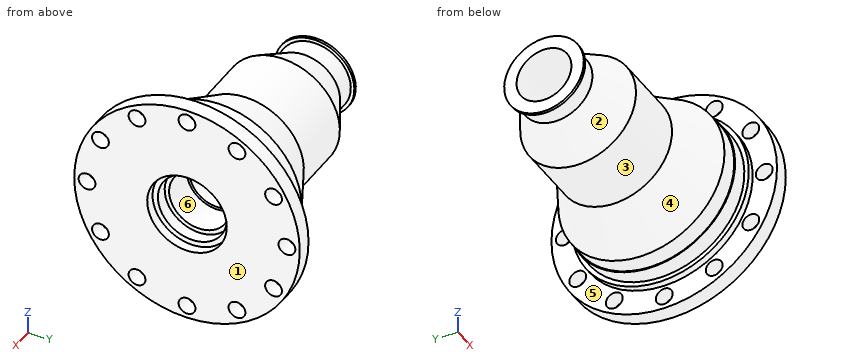
```python
from build123d import *

# Parameters (mm, degrees)
SKETCH_3_R           = 9.5
CUT_EXTRUDE_1_DEPTH  = 321.526909947
SKETCH_4_R           = 9.5
CUT_EXTRUDE_2_DEPTH  = 321.526909947
SKETCH_5_R           = 9.5
CUT_EXTRUDE_3_DEPTH  = 321.526909947
SKETCH_6_R           = 9.5
CUT_EXTRUDE_4_DEPTH  = 321.526909947
SKETCH_7_R           = 9.5
CUT_EXTRUDE_5_DEPTH  = 321.526909947
SKETCH_8_R           = 9.5
CUT_EXTRUDE_6_DEPTH  = 321.526909947
SKETCH_9_R           = 9.5
CUT_EXTRUDE_7_DEPTH  = 321.526909947
SKETCH_10_R          = 9.5
CUT_EXTRUDE_8_DEPTH  = 321.526909947
SKETCH_11_R          = 9.5
CUT_EXTRUDE_9_DEPTH  = 321.526909947
SKETCH_12_R          = 9.5
CUT_EXTRUDE_10_DEPTH = 321.526909947
SKETCH_13_R          = 9.5
CUT_EXTRUDE_11_DEPTH = 321.526909947
SKETCH_14_R          = 9.5
CUT_EXTRUDE_12_DEPTH = 321.526909947


with BuildPart() as part:
    # Эскиз1 → Повернуть1 (revolve)
    with BuildSketch(Plane.XY, mode=Mode.PRIVATE) as revolve_1_sk:
        Polygon((0, 0), (265, 0), (265, 127.5), (247, 127.5), (247, 100), (239, 100), (239, 95), (220, 95), (220, 94), (200, 94), (144, 65.5), (70, 65.5), (25, 41), (3, 41), (3, 45), (0, 45), align=None)
    revolve(revolve_1_sk.sketch.rotate(Axis((0, 0, 0), (1, 0, 0)), 90), axis=Axis((0, 0, 0), (1, 0, 0)))

    # Эскиз2 → Вырез-Повернуть1 (revolve, cut)
    with BuildSketch(Plane.XY, mode=Mode.PRIVATE) as cut_revolve_1_sk:
        Polygon((0, 0), (265, 0), (265, 45), (254, 45), (254, 39), (240, 39), (240, 34), (203.5, 34), (203.5, 31), (0, 31), align=None)
    revolve(cut_revolve_1_sk.sketch.rotate(Axis((0, 0, 0), (1, 0, 0)), 90), axis=Axis((0, 0, 0), (1, 0, 0)), mode=Mode.SUBTRACT)

    # Эскиз3 → Вырез-Вытянуть1 (cut, through all)
    with BuildSketch(Plane(origin=(0, 0, 0), x_dir=(0, 0, -1), z_dir=(1, 0, 0))):
        with Locations((0, 113)):
            Circle(SKETCH_3_R)
    extrude(amount=CUT_EXTRUDE_1_DEPTH, mode=Mode.SUBTRACT)

    # Эскиз4 → Вырез-Вытянуть2 (cut, through all)
    with BuildSketch(Plane(origin=(0, 0, 0), x_dir=(0, 0, -1), z_dir=(1, 0, 0))):
        with Locations((-56.5, 97.860870628)):
            Circle(SKETCH_4_R)
    extrude(amount=CUT_EXTRUDE_2_DEPTH, mode=Mode.SUBTRACT)

    # Эскиз5 → Вырез-Вытянуть3 (cut, through all)
    with BuildSketch(Plane(origin=(0, 0, 0), x_dir=(0, 0, -1), z_dir=(1, 0, 0))):
        with Locations((-97.860870628, 56.5)):
            Circle(SKETCH_5_R)
    extrude(amount=CUT_EXTRUDE_3_DEPTH, mode=Mode.SUBTRACT)

    # Эскиз6 → Вырез-Вытянуть4 (cut, through all)
    with BuildSketch(Plane(origin=(0, 0, 0), x_dir=(0, 0, -1), z_dir=(1, 0, 0))):
        with Locations((-113, 0)):
            Circle(SKETCH_6_R)
    extrude(amount=CUT_EXTRUDE_4_DEPTH, mode=Mode.SUBTRACT)

    # Эскиз7 → Вырез-Вытянуть5 (cut, through all)
    with BuildSketch(Plane(origin=(0, 0, 0), x_dir=(0, 0, -1), z_dir=(1, 0, 0))):
        with Locations((-97.860870628, -56.5)):
            Circle(SKETCH_7_R)
    extrude(amount=CUT_EXTRUDE_5_DEPTH, mode=Mode.SUBTRACT)

    # Эскиз8 → Вырез-Вытянуть6 (cut, through all)
    with BuildSketch(Plane(origin=(0, 0, 0), x_dir=(0, 0, -1), z_dir=(1, 0, 0))):
        with Locations((-56.5, -97.860870628)):
            Circle(SKETCH_8_R)
    extrude(amount=CUT_EXTRUDE_6_DEPTH, mode=Mode.SUBTRACT)

    # Эскиз9 → Вырез-Вытянуть7 (cut, through all)
    with BuildSketch(Plane(origin=(0, 0, 0), x_dir=(0, 0, -1), z_dir=(1, 0, 0))):
        with Locations((0, -113)):
            Circle(SKETCH_9_R)
    extrude(amount=CUT_EXTRUDE_7_DEPTH, mode=Mode.SUBTRACT)

    # Эскиз10 → Вырез-Вытянуть8 (cut, through all)
    with BuildSketch(Plane(origin=(0, 0, 0), x_dir=(0, 0, -1), z_dir=(1, 0, 0))):
        with Locations((56.5, -97.860870628)):
            Circle(SKETCH_10_R)
    extrude(amount=CUT_EXTRUDE_8_DEPTH, mode=Mode.SUBTRACT)

    # Эскиз11 → Вырез-Вытянуть9 (cut, through all)
    with BuildSketch(Plane(origin=(0, 0, 0), x_dir=(0, 0, -1), z_dir=(1, 0, 0))):
        with Locations((97.860870628, -56.5)):
            Circle(SKETCH_11_R)
    extrude(amount=CUT_EXTRUDE_9_DEPTH, mode=Mode.SUBTRACT)

    # Эскиз12 → Вырез-Вытянуть10 (cut, through all)
    with BuildSketch(Plane(origin=(0, 0, 0), x_dir=(0, 0, -1), z_dir=(1, 0, 0))):
        with Locations((113, 0)):
            Circle(SKETCH_12_R)
    extrude(amount=CUT_EXTRUDE_10_DEPTH, mode=Mode.SUBTRACT)

    # Эскиз13 → Вырез-Вытянуть11 (cut, through all)
    with BuildSketch(Plane(origin=(0, 0, 0), x_dir=(0, 0, -1), z_dir=(1, 0, 0))):
        with Locations((97.860870628, 56.5)):
            Circle(SKETCH_13_R)
    extrude(amount=CUT_EXTRUDE_11_DEPTH, mode=Mode.SUBTRACT)

    # Эскиз14 → Вырез-Вытянуть12 (cut, through all)
    with BuildSketch(Plane(origin=(0, 0, 0), x_dir=(0, 0, -1), z_dir=(1, 0, 0))):
        with Locations((56.5, 97.860870628)):
            Circle(SKETCH_14_R)
    extrude(amount=CUT_EXTRUDE_12_DEPTH, mode=Mode.SUBTRACT)


solid = part.part
```
The model under review builds one solid part; all positions refer to its coordinate system, in mm. Face numbers are marked on the shaded views. A direction names the side the tool comes from. Give positions to 0.01 mm unless a question says otherwise; leave off trailing zeros. Write each loop counter-clockwise with the first axis right and the second up, starting at its lowest first coordinate (ties: lowest second). Pieces come first, ordered by that corner, then holes.
(1) For P1, Ø1, axis at y = 44.5, z = 76, coming from the -X side; P2, Ø15, axis at y = -113, z = 0, coming from the -X side; P3, Ø8, axis at x = 155.5, y = -7, coming from the +Z side; P4, Ø22, axis at y = 113, z = 0, coming from the -X side, all flat-tipped, find the tip position at first contact; note any pin that passes through.
(2) To check wall thickness, follow L1, parallel to Y at x = 258, z = 0; L2, parallel to Y at x = 252, z = 93.5; L3, parallel to Y at x = 255, z = -56. State the ranges of each line that lie inside material, in increasing order.
(3) Consider section C-C, the plane x = 91.5. Give the boundary of the cut face in (y, z).
(4) Consider section D-D, the plane y = 0. Give the number of separate pieces and of enclosed holes in the cut face, and give its area (3 significant figures).
(5) Tool access review of the marked faces 1, 2 and 3: name each direction out of +Z, -Z, +X, -X, +Y, -Y from which nothing blocks a thin tool from reaching the whole face with its end or side.
(6) The part is to be moulded in two halves that separate along Z. For the marked faces 4, 5 and 6, say which applies: released by +Z, released by -Z, zero draft, split by the parting line, or undercut.
(7) Consider section A-A, the plane y = -113. Give the boundary of the cut face in (x, z), and give its area (3 significant figures).
Returned:
1. P1: stops at x = 187.36
1. P2: passes through
1. P3: stops at z = 73.09
1. P4: stops at x = 247
2. L1: y = -127.5 to -122.5, -103.5 to -45, 45 to 103.5, 122.5 to 127.5
2. L2: y = -86.68 to -64.94, -48.06 to 48.06, 64.94 to 86.68
2. L3: y = -114.54 to -107.35, -88.37 to 88.37, 107.35 to 114.54
3. outline: circle Ø131 at (0, 0); hole circle Ø62 at (0, 0)
4. separate pieces: 4
4. enclosed holes: 0
4. area: 21,200 mm2
5. face 1: +Z, -Z, +X, +Y, -Y
5. face 2: none
5. face 3: -X
6. face 4: split by the parting line
6. face 5: zero draft
6. face 6: undercut
7. outline: (247, -59.05) - (265, -59.05) - (265, -9.5) - (247, -9.5) - close; (247, 9.5) - (265, 9.5) - (265, 59.05) - (247, 59.05) - close
7. area: 1,780 mm2
